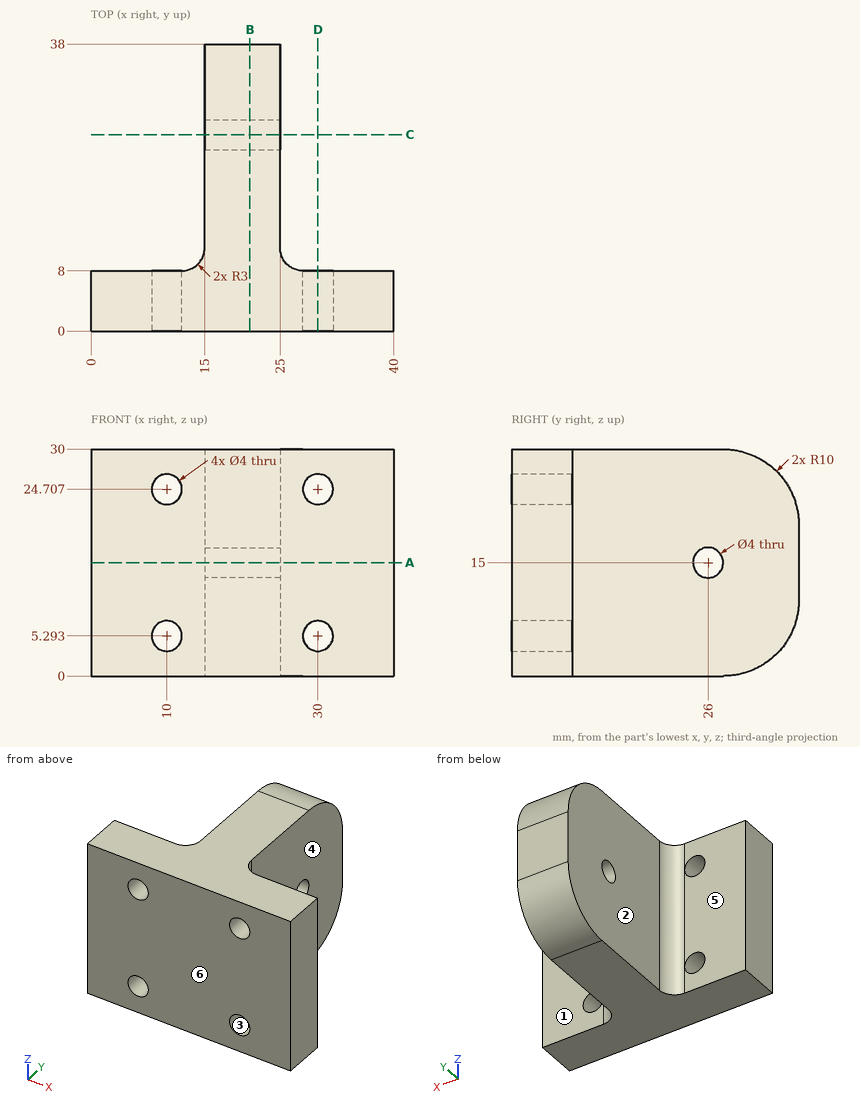
Part print with two shaded views. Sizes in mm from the minimum x, y, z corner. A direction names the side the tool comes from. Round coordinates to 2 decimals unless told otherwise and drop trailing zeros. Write each loop counter-clockwise with the first axis right and the second up, starting at its lowest first coordinate (ties: lowest second). Pieces come first, ordered by that corner, then holes. Notation, with made-up numbers: (-11, 80.25) - (23, 80.25) arc R27 cw to (23, 108.25) - close; hole circle Ø8 at (70, -35.5). An arc over 180 degrees is marked (long way). Answer as CSV lines item,"result".
Q1. Cut at A-A (z = 15). Write the cut outline in (x, y).
Report:
outline,"(0, 0) - (40, 0) - (40, 8) - (28, 8) arc R3 cw to (25, 11) - (25, 24) - (15, 24) - (15, 11) arc R3 cw to (12, 8) - (0, 8) - close; (15, 28) - (25, 28) - (25, 38) - (15, 38) - close"
Q2. Cut at D-D (x = 30). Write the cut outline in (y, z), and give its area (3 significant figures).
Report:
outline,"(0, 0) - (8, 0) - (8, 3.29) - (0, 3.29) - close; (0, 7.29) - (8, 7.29) - (8, 22.71) - (0, 22.71) - close; (0, 26.71) - (8, 26.71) - (8, 30) - (0, 30) - close"
area,"176 mm^2"
Q3. Cut at B-B (x = 21). Write the cut outline in (y, z).
Report:
outline,"(0, 0) - (28, 0) arc R10 ccw to (38, 10) - (38, 20) arc R10 ccw to (28, 30) - (0, 30) - close; hole circle Ø4 at (26, 15)"
Q4. Pull direction X, two halves, no side cores. Call the marked faces 1, 2, 3 and 4: +X half, -X half, draft (parallel to the pull), parting line (faces both ways), or undercut.
Report:
face 1,"draft"
face 2,"-X half"
face 3,"undercut"
face 4,"+X half"
Q5. Drill centre lines: probe 1 along Z at (x, y) = (30, 4.25); probe 2 along Z at (x, y) = (30.5, 5.5); probe 3 along X at (y, z) = (16.5, 5). Where is each one in solid material? Low to high. Write a range as [from, to].
Report:
probe 1,"z = [0, 3.29], [7.29, 22.71], [26.71, 30]"
probe 2,"z = [0, 3.36], [7.23, 22.77], [26.64, 30]"
probe 3,"x = [15, 25]"
Q6. Drop flat-ended pins along their axis: pin 1 (3 mm diameter, centred on x = 15, y = 29.5, fed in from +Z); pin 2 (8 mm diameter, centred on x = 7, z = 16.5, fed in from +Y); pin 3 (2 mm diameter, centred on x = 27.5, z = 21, fed in from +Y); pin 4 (6.5 mm diameter, centred on x = 10, z = 5.29, fed in from +Y). Give the stop position or say it passes through.
Report:
pin 1,"stops at z = 30"
pin 2,"stops at y = 8"
pin 3,"stops at y = 8.4"
pin 4,"stops at y = 8.27"
Q7. Cut at C-C (y = 26). Write the cut outline in (x, z).
Report:
outline,"(15, 0) - (25, 0) - (25, 13) - (15, 13) - close; (15, 17) - (25, 17) - (25, 30) - (15, 30) - close"
Q8. Tool access for the marked faces 5 and 6: list every direction of +Z, -Z, +X, -X, +Y, -Y with a clear straight run to the whole face (end or side of a thin tool).
Report:
face 5,"+Z, -Z, -X, +Y"
face 6,"+Z, -Z, +X, -X, -Y"
